For this review, take the finished solid that the model builds, in its own axes (mm). Face numbers are marked on the shaded views. A direction names the side the tool comes from. Coordinates: 2 decimals unless noted, no trailing zeros. Order: outer loops, then holes, each group sorted by start corner. A loop starts at its lowest first (then second) coordinate and runs counter-clockwise, first axis right, second up. Notation, with made-up numbers: (-18, -37.5) -> (31, -37.5) arc R22 cw to (31, -10.5) -> close; hole circle Ø4 at (79.25, 57). An arc over 180 degrees is marked (long way). Return JSON: item names as keys, results as strings. Group by question number.
Item 1: For line 1 along X through (y, z) = (38.5, -168); line 2 along Y through (x, z) = (0, 301.9); line 3 along X through (y, z) = (42, -280), list the stretches that pass through material, from the lowest coordinate up.
Item 2: Draft analysis for pull direction Z (two halves, no side actions). For the marked faces 3, 4 and 5, state which applies: +Z half, -Z half, draft (parallel to the pull), parting line (faces both ways), or undercut.
Item 3: Take a section at C-C (y = -30). Write out the cut boundary in (x, z).
Item 4: Take a section at B-B (x = 210). Write out the cut boundary in (y, z).
Item 5: Insertion check: pin 1 (6 mm diameter, centred on x = 161, z = -190, fed in from -Y); pin 2 (19 mm diameter, centred on x = 0, y = 0, fed in from +Z). Each pin has a flat end and moves straight along its axis. Give the tip position at first contact, or say it passes through.
Item 6: Take a section at A-A (z = -280). Write out the cut boundary in (x, y).
Item 7: Take a section at D-D (x = 26). Write out the cut boundary in (y, z).
Item 8: Machinability: for the marked faces 1 and 2, which of the approach directions +Z, -Z, +X, -X, +Y, -Y give a long, thin tool a straight path to every point of the face, cutting with its end or side? Answer none if there is none.
```python
from build123d import *

# Parameters (mm, degrees)
SKETCH1_W           = 520
SKETCH1_H           = 610
BOSS_EXTRUDE1_DEPTH = 45
SHELL1_T            = -5
SKETCH4_R           = 10.5
CUT_EXTRUDE2_DEPTH  = 10
SKETCH5_R           = 10.5
CUT_EXTRUDE3_DEPTH  = 10
SKETCH3_R           = 36.5
CUT_EXTRUDE4_DEPTH  = 25


with BuildPart() as part:
    # Sketch1 → Boss-Extrude1 (new, symmetric)
    with BuildSketch(Plane(origin=(0, 0, 0), x_dir=(1, 0, 0), z_dir=(0, 1, 0))):
        Rectangle(SKETCH1_W, SKETCH1_H)
    extrude(amount=BOSS_EXTRUDE1_DEPTH, both=True)

    # Shell1
    shell1_openings = [part.faces().sort_by_distance(p)[0] for p in [
        (0, -45, 0),
    ]]
    offset(amount=SHELL1_T, openings=shell1_openings, kind=Kind.INTERSECTION)

    # Sketch4 → Cut-Extrude2 (cut)
    with BuildSketch(Plane(origin=(0, 45, 0), x_dir=(1, 0, 0), z_dir=(0, 1, 0))):
        with Locations(Location((0, 280, 0), (0, 0, 270))):
            Circle(SKETCH4_R)
    extrude(amount=-CUT_EXTRUDE2_DEPTH, mode=Mode.SUBTRACT)

    # Sketch5 → Cut-Extrude3 (cut)
    with BuildSketch(Plane.XY.offset(305)):
        Circle(SKETCH5_R)
    extrude(amount=-CUT_EXTRUDE3_DEPTH, mode=Mode.SUBTRACT)

    # Sketch3 → Cut-Extrude4 (cut)
    with BuildSketch(Plane.XY.offset(305)):
        with Locations((-210, 0)):
            Circle(SKETCH3_R)
        with Locations(Location((210, 0, 0), (0, 0, 180))):
            Circle(SKETCH3_R)
    extrude(amount=-CUT_EXTRUDE4_DEPTH, mode=Mode.SUBTRACT)


solid = part.part
```
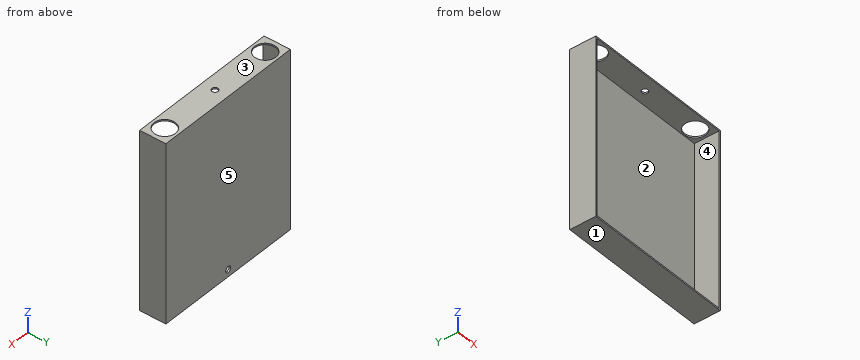
Findings below:
{
 "1": {"line 1": "x = -260 to -255, 255 to 260", "line 2": "y = -45 to -10.5, 10.5 to 45", "line 3": "x = -260 to -10.5, 10.5 to 260"},
 "2": {"face 3": "+Z half", "face 4": "undercut", "face 5": "draft"},
 "3": {"outline": "(-260, -305) -> (260, -305) -> (260, 305) -> (230.79, 305) -> (230.79, 300) -> (255, 300) -> (255, -300) -> (-255, -300) -> (-255, 300) -> (-230.79, 300) -> (-230.79, 305) -> (-260, 305) -> close; (-189.21, 300) -> (189.21, 300) -> (189.21, 305) -> (-189.21, 305) -> close"},
 "4": {"outline": "(-45, -305) -> (45, -305) -> (45, 305) -> (36.5, 305) -> (36.5, 300) -> (40, 300) -> (40, -300) -> (-45, -300) -> close; (-45, 300) -> (-36.5, 300) -> (-36.5, 305) -> (-45, 305) -> close"},
 "5": {"pin 1": "stops at y = 40", "pin 2": "stops at z = -300"},
 "6": {"outline": "(-260, -45) -> (-255, -45) -> (-255, 40) -> (-10.5, 40) -> (-10.5, 45) -> (-260, 45) -> close; (10.5, 40) -> (255, 40) -> (255, -45) -> (260, -45) -> (260, 45) -> (10.5, 45) -> close"},
 "7": {"outline": "(-45, -305) -> (45, -305) -> (45, 305) -> (-45, 305) -> (-45, 300) -> (40, 300) -> (40, -300) -> (-45, -300) -> close"},
 "8": {"face 1": "-Z, +X, -X, +Y, -Y", "face 2": "-Y"}
}
